Part model, mm, in its own coordinate system. A direction names the side the tool comes from. Round coordinates to 2 decimals unless told otherwise and drop trailing zeros. Loops run counter-clockwise (first coordinate to the right, second up) from the corner with the lowest first, then second, coordinate; pieces in that order, holes last. Notation, with made-up numbers: M 57,-39 L 114,-39 A25 ccw 114,0 Z; hole C 27,-39.5 d11. An arc over 180 degrees is marked long. Answer as CSV lines item,"result". Start each with the question number.
Item 1: Band-saw the part on A-A (y = -9.5). Give the cut face in (x, z), and give its area (3 significant figures).
Item 2: Band-saw the part on B-B (x = 11.25). Give the cut face in (y, z).
Item 3: Drop flat-ended pins along their axis: pin 1 Ø2.5 at (y, z) = (10.5, 0.5) entering from +X; pin 2 Ø3 at (y, z) = (-11.25, 0) entering from -X; pin 3 Ø1.2 at (x, z) = (-11.5, -0.5) entering from -Y. Give the stop position or say it passes through.
Item 4: Band-saw the part on C-C (z = 0). Count the separate pieces of the cut face and the enclosed holes in it, and give its area (3 significant figures).
Item 5: Wall check: line 1 (Y direction, x = 15.05, z = 0); line 2 (Y direction, x = -16, z = -1.6). Give the ranges that are in metal, low to high.
Item 6: Which spindle directions (+Z, -Z, +X, -X, +Y, -Y) get a long thin tool onto all of the face, cutting with end or side? Do faces 4 (the flat face through (-13.75, 11, 0)), 5 (the cylindrical face through (7.16, -10.985, -0.035)), 6 (the cylindrical face through (14.982, 10.881, -1.173)), 7 (the flat face through (11, -13.75, 0)), 8 (the flat face through (16.25, 13, 0)). Say none if no direction does.
Item 7: Mould opens along X. For faces 1 (the flat face through (0, -18.25, 0)), 2 (the cylindrical face through (-12.081, -14.982, 0.906)), 3 (the cylindrical face through (-15.2, 7.3, 0)) say: pulls with the +X half, pulls with the -X half, needs draft (parallel to the pull), parting line crosses it, or undercut.
Autodesk Inventor part; units mm, degrees
ref_plane "YZ Plane" through (0, 0, 0) normal (1, 0, 0) x (0, 1, 0)
ref_plane "XZ Plane" through (0, 0, 0) normal (0, 1, 0) x (-1, 0, 0)
ref_plane "XY Plane" through (0, 0, 0) normal (0, 0, 1) x (1, 0, 0)
sketch "スケッチ1" plane through (0, 0, 0) normal (0, 0, 1) x (1, 0, 0)
  line L0 (-16.25, -16.25) -> (16.25, -16.25) construction
  line L1 (16.25, -16.25) -> (16.25, 16.25) construction
  line L2 (16.25, 16.25) -> (-16.25, 16.25) construction
  line L3 (-16.25, 16.25) -> (-16.25, -16.25) construction
  line L4 (-16.25, -16.25) -> (16.25, 16.25) construction
  line L5 (16.25, -16.25) -> (-16.25, 16.25) construction
  line L6 (-8.35, 16.25) -> (-16.25, 16.25)
  line L7 (-16.25, 16.25) -> (-16.25, 8.35)
  line L8 (8.35, 16.25) -> (16.25, 16.25)
  line L9 (16.25, 16.25) -> (16.25, 8.35)
  line L10 (-16.25, -8.35) -> (-16.25, -16.25)
  line L11 (-16.25, -16.25) -> (-8.35, -16.25)
  line L12 (8.35, -16.25) -> (16.25, -16.25)
  line L13 (16.25, -16.25) -> (16.25, -8.35)
  line L14 (-6.25, 16.25) -> (-6.25, 18.25)
  line L15 (-6.25, 18.25) -> (6.25, 18.25)
  line L16 (6.25, 18.25) -> (6.25, 16.25)
  arc A0 (-8.35, 16.25) -> (-6.25, 16.25) centre (-7.3, 16.25) ccw
  arc A1 (6.25, 16.25) -> (8.35, 16.25) centre (7.3, 16.25) ccw
  line L17 (0, 16.25) -> (0, 0) construction
  line L18 (0, 0) -> (16.25, 0) construction
  line L19 (-16.25, 6.25) -> (-18.25, 6.25)
  line L20 (-18.25, 6.25) -> (-18.25, -6.25)
  line L21 (-18.25, -6.25) -> (-16.25, -6.25)
  arc A2 (-16.25, 6.25) -> (-16.25, 8.35) centre (-16.25, 7.3) ccw
  arc A3 (-16.25, -8.35) -> (-16.25, -6.25) centre (-16.25, -7.3) ccw
  line L22 (-6.25, -16.25) -> (-6.25, -18.25)
  line L23 (-6.25, -18.25) -> (6.25, -18.25)
  line L24 (6.25, -18.25) -> (6.25, -16.25)
  arc A4 (-6.25, -16.25) -> (-8.35, -16.25) centre (-7.3, -16.25) ccw
  arc A5 (8.35, -16.25) -> (6.25, -16.25) centre (7.3, -16.25) ccw
  line L25 (16.25, 6.25) -> (18.25, 6.25)
  line L26 (18.25, 6.25) -> (18.25, -6.25)
  line L27 (18.25, -6.25) -> (16.25, -6.25)
  arc A6 (16.25, 8.35) -> (16.25, 6.25) centre (16.25, 7.3) ccw
  arc A7 (16.25, -6.25) -> (16.25, -8.35) centre (16.25, -7.3) ccw
  line L28 (-12.8, 16.25) -> (-9.7, 16.25) construction
  line L29 (-9.7, 16.25) -> (-9.7, 13.25) construction
  line L30 (-9.7, 13.25) -> (-12.8, 13.25) construction
  line L31 (-12.8, 13.25) -> (-12.8, 16.25) construction
  line L32 (-16.25, 12.8) -> (-13.25, 12.8) construction
  line L33 (-13.25, 12.8) -> (-13.25, 9.7) construction
  line L34 (-13.25, 9.7) -> (-16.25, 9.7) construction
  line L35 (-16.25, 9.7) -> (-16.25, 12.8) construction
  line L36 (-10.1287, 12.25) -> (10.1287, 12.25)
  line L37 (10.1287, 12.25) -> (0, 2.1213)
  line L38 (0, 2.1213) -> (-10.1287, 12.25)
  line L39 (-12.25, 10.1287) -> (-12.25, -10.1287)
  line L40 (-12.25, -10.1287) -> (-2.1213, 0)
  line L41 (-2.1213, 0) -> (-12.25, 10.1287)
  line L42 (-10.1287, -12.25) -> (10.1287, -12.25)
  line L43 (10.1287, -12.25) -> (0, -2.1213)
  line L44 (0, -2.1213) -> (-10.1287, -12.25)
  line L45 (12.25, 10.1287) -> (12.25, -10.1287)
  line L46 (12.25, -10.1287) -> (2.1213, 0)
  line L47 (2.1213, 0) -> (12.25, 10.1287)
  line L48 (-11.25, 16.25) -> (-11.25, 13.25) construction
  line L49 (-13.25, 11.25) -> (-16.25, 11.25) construction
  dimension "d0" = 32.5
  dimension "d1" = 1.05
  dimension "d2" = 2
  dimension "d3" = 10
  dimension "d4" = 3.1
  dimension "d6" = 3
  dimension "d8" = 3
  dimension "d9" = 3
  dimension "d10" = 3
  dimension "d11" = 3
  dimension "d12" = 3
  dimension "d13" = 4
  dimension "d17" = 5
  dimension "d18" = 5
extrude "押し出し1" add sketch "スケッチ1" along normal blind 2.5
mirror "ミラー1" about plane through (0, 0, 0) normal (0, 0, -1) of "押し出し1"
sketch "スケッチ2" plane through (-16.25, -16.25, 2.5) normal (0, -1, 0) x (1, 0, 0)
  line L0 (0, -5) -> (0, 0)
  line L1 (10, 0) -> (22.5, 0) construction
  line L2 (16.25, 0) -> (16.25, -5) construction
  point P0 (16.25, -2.5)
  point P1 (5, -2.5)
  point P2 (27.5, -2.5)
  point P3 (0, -2.5)
  dimension "d19" = 5
hole "穴1" at (-11.25, -16.25, 0) at (11.25, -16.25, 0) direction (0, 1, 0) diameter 2.459 depth 2.5
pattern_circular "円形状パターン1" count 4 over 360 about axis through (0, 0, -10) along (0, 0, 1) of "穴1"
fillet "フィレット1" radius 2 12 edges at (12.25, 10.1287, 0) (12.25, -10.1287, 0) (10.1287, -12.25, 0) (0, 2.1213, 0) (-2.1213, 0, 0) (-10.1287, -12.25, 0) (-12.25, -10.1287, 0) (10.1287, 12.25, 0) (-12.25, 10.1287, 0) (-10.1287, 12.25, 0) (0, -2.1213, 0) (2.1213, 0, 0)
equation "\"d8\" = d6"
equation "\"d10\" = d9"
equation "\"d11\" = d10"
equation "\"d12\" = d11"
equation "\"d18\" = d17"
properties part number "上腕_メインフレーム_1_1" material "アセタール樹脂、黒"
Answer block:
1,outline,"M -16.25,-2.5 L -7.15,-2.5 L -7.15,2.5 L -16.25,2.5 Z; M 7.15,-2.5 L 16.25,-2.5 L 16.25,2.5 L 7.15,2.5 Z"
1,area,"91.0 mm^2"
2,outline,"M -16.25,-2.5 L -7.03,-2.5 L -7.03,2.5 L -16.25,2.5 L -16.25,1.23 L -13.75,1.23 L -13.75,-1.23 L -16.25,-1.23 Z; M 7.03,-2.5 L 16.25,-2.5 L 16.25,-1.23 L 13.75,-1.23 L 13.75,1.23 L 16.25,1.23 L 16.25,2.5 L 7.03,2.5 Z"
3,pin 1,"stops at x = 16.25"
3,pin 2,"stops at x = -16.25"
3,pin 3,"stops at y = -13.75"
4,separate pieces,"1"
4,enclosed holes,"4"
4,area,"726 mm^2"
5,line 1,"y = -16.25 to -12.48, -10.02 to 10.02, 12.48 to 16.25"
5,line 2,"y = -16.25 to -8.32, -6.28 to 6.28, 8.32 to 16.25"
6,face 4,"-X"
6,face 5,"+Z, -Z"
6,face 6,"+X"
6,face 7,"-Y"
6,face 8,"+Z, -Z, +X, +Y"
7,face 1,"needs draft"
7,face 2,"undercut"
7,face 3,"pulls with the -X half"
